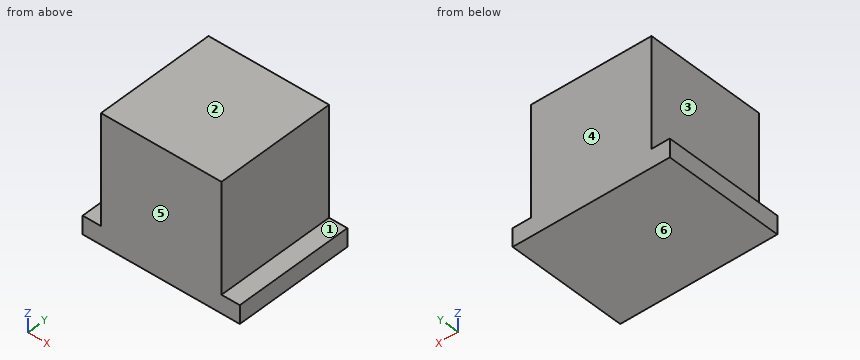
from build123d import *

# Parameters (mm, degrees)
BOX085_W               = 3.5
BOX085_H               = 2.5
BOX085_DEPTH           = 4.5
BOX083_W               = 6.6
BOX083_H               = 8.6
BOX083_DEPTH           = 1
BOX084_W               = 6.6
BOX084_H               = 6.6
BOX084_DEPTH           = 7
CUT022_PLACEMENT_ANGLE = 90


with BuildPart() as sub_cap:
    # Box085 → Box085 (new body)
    with BuildSketch(Plane(origin=(-1.75, -1.25, 0), x_dir=(1, 0, 0), z_dir=(0, 0, 1))):
        with Locations((1.75, 1.25)):
            Rectangle(BOX085_W, BOX085_H)
    extrude(amount=BOX085_DEPTH)


with BuildPart() as cap:
    # Box083 → Box083 (new body)
    with BuildSketch(Plane(origin=(-3.3, -4.3, 11), x_dir=(1, 0, 0), z_dir=(0, 0, 1))):
        with Locations((3.3, 4.3)):
            Rectangle(BOX083_W, BOX083_H)
    extrude(amount=BOX083_DEPTH)


with BuildPart() as switch_cap_master:
    # Box084 → Box084 (new body)
    with BuildSketch(Plane(origin=(-3.3, -3.3, 11), x_dir=(1, 0, 0), z_dir=(0, 0, 1))):
        with Locations((3.3, 3.3)):
            Rectangle(BOX084_W, BOX084_H)
    extrude(amount=BOX084_DEPTH)

    # Fusion023: union cap
    add(cap.part)

    # Cut022: cut sub cap
    add(sub_cap.part, mode=Mode.SUBTRACT)


with BuildPart() as switch_cap_master_1:
    # Cut022 placement: moved
    add(switch_cap_master.part.rotate(Axis((0, 0, 0), (0, 0, -1)), CUT022_PLACEMENT_ANGLE))


solid = switch_cap_master_1.part
Could you check a few things on this model? Use its own coordinates, in mm. Face numbers are marked on the shaded views. A direction names the side the tool comes from. Give positions to 0.01 mm unless a question says otherwise; leave off trailing zeros. Order: outer loops, then holes, each group sorted by start corner. A loop starts at its lowest first (then second) coordinate and runs counter-clockwise, first axis right, second up. Notation, with made-up numbers: (-4, -31) - (40, -31) arc R34 cw to (40, 6) - close; hole circle Ø10 at (-8, 29). An arc over 180 degrees is marked (long way). One line per question, with ' | ' between items. Start each with the question number.
Item 1: I want a section at B-B on z = 16.75. Write out the boundary of the cut face in (x, y).
Item 2: Thinking about a two-plate mould opening in Y: for the marked faces 4, 5 and 6, which applies, pulls with the +Y half, pulls with the -Y half, needs draft (parallel to the pull), parting line crosses it, or undercut?
Item 3: I want a section at C-C on x = 3.5. Write out the boundary of the cut face in (y, z), then the cut area to 3 significant figures.
Item 4: I need wall thicknesses on probe 1 along Z at (x, y) = (3.75, 0.5); probe 2 along X at (y, z) = (-1.25, 16.25). Which ranges of each line are inside material? Lowest first, please. Write a range as [from, to].
Item 5: For the marked faces 1, 2 and 3, which set-ups out of +Z, -Z, +X, -X, +Y, -Y let a thin tool reach every point of the face, with its end or its side?
Item 6: I'm going to push a flat-ended pin straight in: pin 1 Ø1.8 at (y, z) = (-1.5, 16) entering from -X. Where does the tip first touch, or does it pass through?
Item 7: I want a section at A-A on y = -2.25. Write out the boundary of the cut face in (x, z).
Verdict:
1) outline: (-3.3, -3.3) - (3.3, -3.3) - (3.3, 3.3) - (-3.3, 3.3) - close
2) face 4: pulls with the +Y half | face 5: pulls with the -Y half | face 6: needs draft
3) outline: (-3.3, 11) - (3.3, 11) - (3.3, 12) - (-3.3, 12) - close | area: 6.60 mm^2
4) probe 1: [11, 12] | probe 2: [-3.3, 3.3]
5) face 1: +Z, +X, +Y, -Y | face 2: +Z, +X, -X, +Y, -Y | face 3: +Z, -X, +Y, -Y
6) pin 1: x = -3.3
7) outline: (-4.3, 11) - (4.3, 11) - (4.3, 12) - (3.3, 12) - (3.3, 18) - (-3.3, 18) - (-3.3, 12) - (-4.3, 12) - close
